Source: CAD feature listing. Evaluate the final solid. Frame: model axes, mm. A direction names the side the tool comes from. Coordinates: 2 decimals unless noted, no trailing zeros. Loops run counter-clockwise (first coordinate to the right, second up) from the corner with the lowest first, then second, coordinate; pieces in that order, holes last. Notation, with made-up numbers: (15.25, 54.25) - (46.25, 54.25) arc R29 ccw to (46.25, 90.25) - close; hole circle Ø6 at (-29.5, 56.25). An arc over 180 degrees is marked (long way). Write item = value, one per line. Start each with the question number.
from build123d import *

# Parameters (mm, degrees)
F0_R      = 6.1
F0_R_2    = 3.3
F1_DEPTH  = 20
F4_DEPTH  = 2
F6_W      = 37
F6_H      = 18
F7_DEPTH  = 22
F8_R      = 8.99999
F9_R      = 8.99999
F10_R     = 8.99999
F12_W     = 2
F12_H     = 13
F13_DEPTH = 8.2
F14_R     = 3.3
F15_DEPTH = 10
F17_DEPTH = 2


# Not quite as in the source:
# - a fillet or chamfer is up to 0.001 mm smaller than in the source, because OpenCascade refuses the exact size


with BuildPart() as f1:
    # F0 (on Front) → F1 (new body)
    with BuildSketch(Plane.XZ):
        Circle(F0_R)
        Circle(F0_R_2, mode=Mode.SUBTRACT)
    extrude(amount=-F1_DEPTH)

    # F2 (on Top) → F3 (revolve)
    with BuildSketch(Plane.XY):
        with BuildLine():
            Line((-18.5, 12.5), (0, 12.5))
            Line((0, 12.5), (0, 23.5))
            Line((0, 23.5), (-13.5, 23.5))
            ThreePointArc((-13.5, 23.5), (-17.0355339059, 22.0355339059), (-18.5, 18.5))
            Line((-18.5, 18.5), (-18.5, 12.5))
        make_face()
    revolve(axis=Axis((0, 18, 0), (0, 1, 0)))

    # F0 (on Front) → F4 (cut)
    with BuildSketch(Plane.XZ):
        Circle(F0_R)
        Circle(F0_R_2, mode=Mode.SUBTRACT)
    extrude(amount=-F4_DEPTH, mode=Mode.SUBTRACT)

    # F6 (on offset) → F7 (join)
    with BuildSketch(Plane.XZ.offset(-12.5)):
        Rectangle(F6_W, F6_H)
    extrude(amount=-F7_DEPTH)

    # F8 (radius 9 in the source; OpenCascade refuses exactly that, so slightly less here)
    f8_edges = [f1.edges().sort_by_distance(p)[0] for p in [
        (-18.5, 23.5, -9),
    ]]
    fillet(f8_edges, radius=F8_R)

    # F9 (radius 9 in the source; OpenCascade refuses exactly that, so slightly less here)
    f9_edges = [f1.edges().sort_by_distance(p)[0] for p in [
        (-18.5, 23.5, 9),
    ]]
    fillet(f9_edges, radius=F9_R)

    # F10 (radius 9 in the source; OpenCascade refuses exactly that, so slightly less here)
    f10_edges = [f1.edges().sort_by_distance(p)[0] for p in [
        (18.5, 23.5, -9),
        (18.5, 23.5, 9),
    ]]
    fillet(f10_edges, radius=F10_R)

    # F12 (on face) → F13 (cut)
    with BuildSketch(Plane.XZ):
        Rectangle(F12_W, F12_H)
    extrude(amount=-F13_DEPTH, mode=Mode.SUBTRACT)

    # F14 (on face) → F15 (cut)
    with BuildSketch(Plane.XZ.offset(-12.5)):
        Circle(F14_R)
    extrude(amount=-F15_DEPTH, mode=Mode.SUBTRACT)

    # F16 (on offset) → F17 (cut)
    with BuildSketch(Plane(origin=(0, 34.5, 0), x_dir=(-1, 0, 0), z_dir=(0, 1, 0))):
        with BuildLine():
            ThreePointArc((16, -1), (17, 0), (16, 1))
            Line((16, 1), (9, 1))
            ThreePointArc((9, 1), (8, 0), (9, -1))
            Line((9, -1), (16, -1))
        make_face()
    extrude(amount=-F17_DEPTH, mode=Mode.SUBTRACT)


solid = f1.part
Item 1: First-contact query: pin 1 (1 mm diameter, centred on x = 6, y = 29, fed in from +Z); pin 2 (3 mm diameter, centred on y = 26, z = -4.5, fed in from +X); pin 3 (1 mm diameter, centred on x = -12.5, y = 33.5, fed in from +Z). Flat tips, straight axial feed; report the tip coordinate or a pass-through.
Item 2: Reachability of faces 1 (the cylindrical face through (-1.322, 7.176, -5.955)), 2 (the flat face through (-1, 5, -5)), 3 (the flat face through (0, 29, 9)) from +Z, -Z, +X, -X, +Y, -Y: full face, straight path, thin tool, end or side. Return the list, or none.
Item 3: Cut plane B-B (x = 0). Return the cut outline in (y, z).
Item 4: Draft query along X for faces 4 (the flat face through (0, 22.5, 0)), 5 (the cylindrical face through (0.407, 15.458, -18.496)), 6 (the flat face through (0, 23.5, 11)). Return one class per face: released by +X, released by -X, zero draft, split by the parting line, or undercut.
Item 5: Material intervals for L1, parallel to X at y = 9.75, z = 0; L2, parallel to X at y = 16.5, z = 0, sorted ascending. Write a range as [from, to].
Responses:
q1.pin_1 = 9
q1.pin_2 = 17.99
q1.pin_3 = 8.65
q2.face_1 = -Y
q2.face_2 = +Z, -Z, -Y
q2.face_3 = +Z, +X, -X, +Y
q3.outline = (8.2, -6.1) - (12.5, -6.1) - (12.5, -18.5) - (18.5, -18.5) arc R5 ccw to (23.5, -13.5) - (23.5, -9) - (34.5, -9) - (34.5, 9) - (23.5, 9) - (23.5, 13.5) arc R5 ccw to (18.5, 18.5) - (12.5, 18.5) - (12.5, 6.1) - (8.2, 6.1) - (8.2, 3.3) - (22.5, 3.3) - (22.5, -3.3) - (8.2, -3.3) - close
q4.face_4 = undercut
q4.face_5 = split by the parting line
q4.face_6 = zero draft
q5.L1 = [-6.1, -3.3], [3.3, 6.1]
q5.L2 = [-18.5, -3.3], [3.3, 18.5]
